For this review, take the finished solid that the model builds, in its own axes (mm). A direction names the side the tool comes from. Coordinates: 2 decimals unless noted, no trailing zeros. Loops run counter-clockwise (first coordinate to the right, second up) from the corner with the lowest first, then second, coordinate; pieces in that order, holes last. Notation, with made-up numbers: (42, 64.5) -> (75, 64.5) arc R26 cw to (75, 88.5) -> close; hole circle Ø7 at (85.5, 53). An arc over 180 degrees is marked (long way). Answer in a Markdown table with one row per item.
from build123d import *

# Parameters (mm, degrees)
PAD_DEPTH       = 22.5
POCKET_DEPTH    = 29
SKETCH002_R     = 1.6
POCKET001_DEPTH = 5
SKETCH003_R     = 1.8
POCKET002_DEPTH = 5
CHAMFER001_SIZE = 4
POCKET003_DEPTH = 7
SKETCH005_W     = 8
SKETCH005_H     = 36.404098
POCKET004_DEPTH = 0.2


with BuildPart() as part:
    # Sketch → Pad (new body, symmetric)
    with BuildSketch(Plane.XZ):
        Polygon((0, 0), (8.4367642811, 0), (8.4367642811, 1.2), (0.4367642811, 1.2), (-12.998966821, 12.4739170124), (-10.5145511425, 26.563738482), (-11.6963204461, 26.7721162952), (-14.3010431111, 12), align=None)
    extrude(amount=PAD_DEPTH, both=True)

    # Sketch001 (on Face7 of Pad) → Pocket (cut)
    with BuildSketch(Plane(origin=(-15.9219347561, 0, 2.8074666826), x_dir=(-0.1736481777, 0, -0.984807753), z_dir=(-0.984807753, 0, 0.1736481777))):
        Polygon((-10, -22.5), (0, -14.1090036882), (0, -23.5), (-10, -23.5), align=None)
        Polygon((-10, 22.5), (0, 14.1090036882), (0, 23.5), (-10, 23.5), align=None)
    extrude(amount=-POCKET_DEPTH, mode=Mode.SUBTRACT)

    # Sketch002 (on Face7 of Pocket) → Pocket001 (cut)
    with BuildSketch(Plane(origin=(0, 0, 1.2), x_dir=(-1, 0, 0), z_dir=(0, 0, 1))):
        with Locations((-4.5, 10)):
            Circle(SKETCH002_R)
        with Locations((-4.5, -10)):
            Circle(SKETCH002_R)
        Polygon((-9.5, -9.5), (-4.5, -4.5), (-4.5, 4.5), (-9.5, 9.5), align=None)
    extrude(amount=-POCKET001_DEPTH, mode=Mode.SUBTRACT)

    # Sketch003 (on Face13 of Pocket001) → Pocket002 (cut)
    with BuildSketch(Plane(origin=(-15.9219347561, 0, 2.8074666826), x_dir=(-0.1736481777, 0, -0.984807753), z_dir=(-0.984807753, 0, 0.1736481777))):
        with Locations((-16, 18)):
            Circle(SKETCH003_R)
        with Locations((-16, -18)):
            Circle(SKETCH003_R)
    extrude(amount=-POCKET002_DEPTH, mode=Mode.SUBTRACT)

    # Chamfer001
    chamfer001_edges = [part.edges().sort_by_distance(p)[0] for p in [
        (-11.105436, -22.5, 26.667927),
        (-11.105436, 22.5, 26.667927),
    ]]
    chamfer(chamfer001_edges, length=CHAMFER001_SIZE)

    # Sketch004 → Pocket003 (cut, symmetric)
    with BuildSketch(Plane(origin=(-5.5127970494, 0, 0), x_dir=(0, 0, 1), z_dir=(1, 0, 0))):
        Polygon((1.4, 6.5), (1.4, -6.5), (4, -11.5), (8, -11.5), (8, 11.5), (4, 11.5), align=None)
    extrude(amount=POCKET003_DEPTH, both=True, mode=Mode.SUBTRACT)

    # Sketch005 (on Face16 of Pocket003) → Pocket004 (cut)
    with BuildSketch(Plane(origin=(0, 0, 1.2), x_dir=(-1, 0, 0), z_dir=(0, 0, 1))):
        with Locations((-4.90745, 0)):
            Rectangle(SKETCH005_W, SKETCH005_H)
    extrude(amount=-POCKET004_DEPTH, mode=Mode.SUBTRACT)


solid = part.part
Item 1: Take a section at A-A, the plane y = 2. State the section outline as (x, z) points, and give its area (3 significant figures).
Worked answers:
| item | result |
|---|---|
| outline | (-14.3, 12) -> (-9.53, 8) -> (-7.67, 8) -> (-13, 12.47) -> (-10.51, 26.56) -> (-11.7, 26.77) -> close; (-1.67, 1.4) -> (0, 0) -> (4.5, 0) -> (4.5, 1) -> (0.91, 1) -> (0.91, 1.2) -> (0.44, 1.2) -> (0.2, 1.4) -> close |
| area | 31.4 mm² |
Item 2: For faces 4 (the flat face through (4.5, 0.1, 0.5)), 5 (the flat face through (-2.2, -9, 2.7)), 6 (the flat face through (-9, 0, 8)), list the 3-axis set-ups (+Z, -Z, +X, -X, +Y, -Y) from which the entire face can be reached by the end or side of a thin tool; tool diameter is ignored.
Worked answers:
| item | result |
|---|---|
| face 4 | +Z, -Z, +X |
| face 5 | +Z, +X, -X |
| face 6 | -Z, +X, -X |
Item 3: Take a section at C-C, the plane y = 10. State the section outline as (x, z) points, and give its area (3 significant figures).
Worked answers:
| item | result |
|---|---|
| outline | (-14.3, 12) -> (-9.53, 8) -> (-7.67, 8) -> (-13, 12.47) -> (-10.51, 26.56) -> (-11.7, 26.77) -> close; (-3.84, 3.22) -> (0, 0) -> (2.9, 0) -> (2.9, 1) -> (0.91, 1) -> (0.91, 1.2) -> (0.44, 1.2) -> (-1.97, 3.22) -> close; (6.1, 0) -> (8.44, 0) -> (8.44, 1) -> (6.1, 1) -> close |
| area | 35.5 mm² |
Item 4: For L1, parallel to Z at x = 2.5, y = 2.5; L2, parallel to X at y = 10, z = 0.4; L3, parallel to X at y = 12.5, z = 8, list the stretches that pass through material, from the lowest coordinate up.
Worked answers:
| item | result |
|---|---|
| L1 | 0 to 1 |
| L2 | -0.48 to 2.9, 6.1 to 8.44 |
| L3 | -9.53 to -7.67 |
Item 5: Take a section at D-D, the plane x = 5. State the section outline as (y, z) points, and give its area (3 significant figures).
Worked answers:
| item | result |
|---|---|
| outline | (-15.66, 1) -> (-14.84, 0) -> (-11.52, 0) -> (-11.52, 1) -> close; (-8.48, 0) -> (-5, 0) -> (-5, 1) -> (-8.48, 1) -> close; (5, 0) -> (8.48, 0) -> (8.48, 1) -> (5, 1) -> close; (11.52, 0) -> (14.84, 0) -> (15.66, 1) -> (11.52, 1) -> close |
| area | 14.4 mm² |
Item 6: The part is to be moulded in two halves that separate along X. For faces 1 (the flat face through (-12.98, -0.32, 19.49)), 2 (the cylindrical face through (4.85, 11.56, 0.51)), 3 (the flat face through (-2.2, 9, 2.7)), say which applies: +X half, -X half, draft (parallel to the pull), parting line (faces both ways), or undercut.
Worked answers:
| item | result |
|---|---|
| face 1 | -X half |
| face 2 | undercut |
| face 3 | draft |
Item 7: Take a section at B-B, the plane x = -6.25. State the section outline as (y, z) points, and give its area (3 significant figures).
Worked answers:
| item | result |
|---|---|
| outline | (-18.83, 6.81) -> (-17.53, 5.24) -> (-11.5, 5.24) -> (-11.5, 6.81) -> close; (11.5, 5.24) -> (17.53, 5.24) -> (18.83, 6.81) -> (11.5, 6.81) -> close |
| area | 20.9 mm² |
Item 8: Insertion check: pin 1 (6 mm diameter, centred on x = -8.5, z = 7, fed in from -Y); pin 2 (8 mm diameter, centred on x = -8, y = -17, fed in from -Z); pin 3 (1 mm diameter, centred on y = -3, z = 15, fed in from +X); pin 4 (5 mm diameter, centred on x = 4.5, y = 10, fed in from -Z). Each pin has a flat end and moves straight along its axis. Give the tip position at first contact, or say it passes through.
Worked answers:
| item | result |
|---|---|
| pin 1 | y = -20.73 |
| pin 2 | z = 3.4 |
| pin 3 | x = -12.47 |
| pin 4 | z = 0 |
